Autodesk Inventor part; units mm, degrees
ref_plane "YZ Plane" through (0, 0, 0) normal (1, 0, 0) x (0, 1, 0)
ref_plane "XZ Plane" through (0, 0, 0) normal (0, 1, 0) x (-1, 0, 0)
ref_plane "XY Plane" through (0, 0, 0) normal (0, 0, 1) x (1, 0, 0)
sketch "Skizze1" plane through (0, 0, 0) normal (0, 0, 1) x (1, 0, 0)
  line L0 (-10, -35) -> (70, -35)
  line L1 (70, -35) -> (70, 50)
  line L2 (70, 50) -> (-10, 50)
  line L3 (-10, 50) -> (-10, -35)
  line L4 (0, 67) -> (0, -52)
  line L5 (-26, 0) -> (86, 0)
  dimension "d0" = 80
  dimension "d1" = 85
  dimension "d4" = 35
  dimension "d5" = 10
extrude "Extrusion1" add sketch "Skizze1" along normal blind 1.6
sketch "Skizze3" plane through (0, 0, 1.6) normal (0, 0, 1) x (1, 0, 0)
  line L0 (-10, -35) -> (70, -35)
  line L1 (70, -35) -> (70, 50)
  line L2 (70, 50) -> (-10, 50)
  line L3 (-10, 50) -> (-10, -35)
  line L4 (-10, -35) -> (0, -35)
  line L5 (0, -35) -> (0, -27)
  line L6 (0, -27) -> (-10, -27)
  line L7 (-10, -27) -> (-10, -35)
  line L8 (70, 50) -> (-10, 50)
  line L9 (-10, 50) -> (16, 50)
  line L10 (16, 50) -> (16, 40)
  line L11 (16, 40) -> (-10, 40)
  line L12 (-10, 40) -> (-10, 50)
  point P0 (0, 0)
  dimension "d19" = 10
  dimension "d20" = 8
  dimension "d23" = 26
  dimension "d24" = 10
extrude "Extrusion2" cut sketch "Skizze3" against normal through all contours L3 L6 L5 L0 | L3 L2 L10 L11
sketch "Skizze2" plane through (0, 0, 1.6) normal (0, 0, 1) x (1, 0, 0)
  line L0 (-26, 0) -> (86, 0)
  line L1 (0, 67) -> (0, -52)
  point P0 (0, 0)
  point P1 (56, 46)
  point P2 (56, -31)
  point P3 (-6, 6)
  dimension "d13" = 56
  dimension "d14" = 46
  dimension "d15" = 6
  dimension "d17" = 31
  dimension "d18" = 56
  dimension "d35" = 6
hole "Montage" at (56, 46, 1.6) at (56, -31, 1.6) at (-6, 6, 1.6) direction (0, 0, -1) diameter 3 end through all
sketch "Skizze4" plane through (0, 0, 1.6) normal (0, 0, 1) x (1, 0, 0)
  line L0 (0, 67) -> (0, -52)
  line L1 (-26, 0) -> (86, 0)
  line L2 (11, -32) -> (11, 24) construction
  point P0 (0, 0)
  dimension "d25" = 11
  dimension "d26" = 32
  dimension "d27" = 56
hole "Display" at (11, 24, 1.6) at (11, -32, 1.6) direction (0, 0, -1) diameter 3.2 end through all
fillet "Rundung1" radius 1 8 edges at (-10, -27, 0.8) (0, -27, 0.8) (0, -35, 0.8) (70, -35, 0.8) (70, 50, 0.8) (16, 50, 0.8) (16, 40, 0.8) (-10, 40, 0.8)
properties part number "Mainboard" material "Phenolharz"
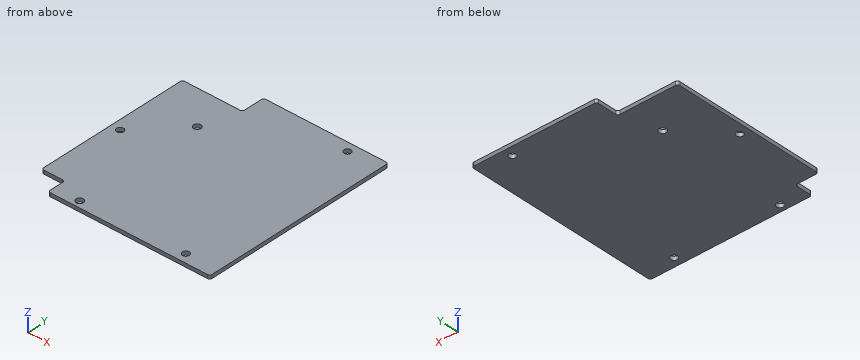
Work out the finished part from the listing and answer in its coordinate system (mm). Give positions to 0.01 mm unless a question says otherwise; leave off trailing zeros. Loops run counter-clockwise (first coordinate to the right, second up) from the corner with the lowest first, then second, coordinate; pieces in that order, holes last. Notation, with made-up numbers: (64, -24) -> (90, -24) arc R23 ccw to (90, 15) -> close; hole circle Ø3 at (86, -1.75). An arc over 180 degrees is marked (long way). Put each result on its own line as item: value. Start each with the question number.
Item 1: The part is cut by section D-D (z = 1.15). Give the vertices of the cut face in (x, y), then the cut area to 3 significant figures.
Item 2: Find the intervals of material crossed by L1, parallel to Y at x = 56, z = 0.7; L2, parallel to Y at x = 11, z = 1.1; L3, parallel to X at y = 24, z = 1, in increasing order. Write a range as [from, to].
Item 3: The part is cut by section C-C (y = 6). Give the vertices of the cut face in (x, z).
Item 4: The part is cut by section B-B (x = -6). Give the vertices of the cut face in (y, z), then the cut area to 3 significant figures.
Item 5: The part is cut by section A-A (x = 11). Give the vertices of the cut face in (y, z).
Item 6: Each of these flat-tipped pins is pushed along its axis until it touches: P1, Ø4, axis at x = 56, y = -31, coming from the +Z side; P2, Ø0.5, axis at y = 44, z = 0.5, coming from the -X side; P3, Ø0.8, axis at x = -7, z = 1, coming from the -Y side; P4, Ø0.8, axis at y = -30, z = 0.5, coming from the -X side. Where does it stop, or does it pass through?
Answers below:
1. outline: (-10, -26) arc R1 ccw to (-9, -27) -> (-1, -27) arc R1 cw to (0, -28) -> (0, -34) arc R1 ccw to (1, -35) -> (69, -35) arc R1 ccw to (70, -34) -> (70, 49) arc R1 ccw to (69, 50) -> (17, 50) arc R1 ccw to (16, 49) -> (16, 41) arc R1 cw to (15, 40) -> (-9, 40) arc R1 ccw to (-10, 39) -> close; hole circle Ø3 at (-6, 6); hole circle Ø3.2 at (11, -32); hole circle Ø3.2 at (11, 24); hole circle Ø3 at (56, -31); hole circle Ø3 at (56, 46)
1. area: 6,420 mm2
2. L1: [-35, -32.5], [-29.5, 44.5], [47.5, 50]
2. L2: [-35, -33.6], [-30.4, 22.4], [25.6, 40]
2. L3: [-10, 9.4], [12.6, 70]
3. outline: (-10, 0) -> (-7.5, 0) -> (-7.5, 1.6) -> (-10, 1.6) -> close; (-4.5, 0) -> (70, 0) -> (70, 1.6) -> (-4.5, 1.6) -> close
4. outline: (-27, 0) -> (4.5, 0) -> (4.5, 1.6) -> (-27, 1.6) -> close; (7.5, 0) -> (40, 0) -> (40, 1.6) -> (7.5, 1.6) -> close
4. area: 102 mm2
5. outline: (-35, 0) -> (-33.6, 0) -> (-33.6, 1.6) -> (-35, 1.6) -> close; (-30.4, 0) -> (22.4, 0) -> (22.4, 1.6) -> (-30.4, 1.6) -> close; (25.6, 0) -> (40, 0) -> (40, 1.6) -> (25.6, 1.6) -> close
6. P1: z = 1.6
6. P2: x = 16
6. P3: y = -27
6. P4: x = 0
